The listing builds one solid part. Answer for the finished solid, in the listing's coordinates (mm). A direction names the side the tool comes from. Round coordinates to 2 decimals unless told otherwise and drop trailing zeros. Order: outer loops, then holes, each group sorted by start corner. A loop starts at its lowest first (then second) coordinate and runs counter-clockwise, first axis right, second up. Notation, with made-up numbers: (-30, 41.5) - (-18, 41.5) arc R19 cw to (-18, 47.5) - close; hole circle Ø2 at (21, -19). An arc over 180 degrees is marked (long way). Write item = value, one per line.
from build123d import *

# Parameters (mm, degrees)
SKETCH_1_R          = 95
EXTRUDE_1_DEPTH     = 50
SKETCH_2_W          = 90
SKETCH_2_H          = 100
EXTRUDE_2_DEPTH     = 150
SKETCH_3_R          = 40
CUT_EXTRUDE_1_DEPTH = 241.935676063
SHELL_1_OUTLINE_R   = 92
SHELL_1_OUTLINE_R_2 = 43
SHELL_1_DEPTH       = 47
SHELL_START         = 47
SHELL_1_2_DEPTH     = 150


# Read off the part's stored shape, not the designer's step: Оболочка1
with BuildPart() as part:
    # Эскиз1 → Бобышка-Вытянуть1 (new body)
    with BuildSketch(Plane.XY):
        Circle(SKETCH_1_R)
    extrude(amount=EXTRUDE_1_DEPTH)

    # Эскиз2 → Бобышка-Вытянуть2 (add)
    with BuildSketch(Plane.XY.offset(50)):
        Rectangle(SKETCH_2_W, SKETCH_2_H)
    extrude(amount=EXTRUDE_2_DEPTH)

    # Эскиз3 → Вырез-Вытянуть1 (cut, through all)
    with BuildSketch(Plane.XY.offset(200)):
        Circle(SKETCH_3_R)
    extrude(amount=-CUT_EXTRUDE_1_DEPTH, mode=Mode.SUBTRACT)

    # Оболочка1 outline → Оболочка1 (cut)
    with BuildSketch(Plane.XY):
        Circle(SHELL_1_OUTLINE_R)
        Circle(SHELL_1_OUTLINE_R_2, mode=Mode.SUBTRACT)
    extrude(amount=SHELL_1_DEPTH, mode=Mode.SUBTRACT)

    # Shell 1 2 outline → Shell 1 2 (cut)
    with BuildSketch(Plane.XY.offset(SHELL_START)):
        with BuildLine():
            ThreePointArc((-42, 9.219544457), (0, 43), (42, 9.219544457))
            Line((42, 9.219544457), (42, 47))
            Line((42, 47), (-42, 47))
            Line((-42, 47), (-42, 9.219544457))
        make_face()
        with BuildLine():
            Line((42, -47), (42, -9.219544457))
            ThreePointArc((42, -9.219544457), (0, -43), (-42, -9.219544457))
            Line((-42, -9.219544457), (-42, -47))
            Line((-42, -47), (42, -47))
        make_face()
    extrude(amount=SHELL_1_2_DEPTH, mode=Mode.SUBTRACT)


solid = part.part
Q1. Flat-ended cylindrical pins translate along their axes: P1, Ø4, axis at x = 50, y = -12, coming from the +Z side; P2, Ø1.5, axis at x = 43.5, z = 86, coming from the +Y side; P3, Ø2, axis at x = -71, y = -37, coming from the -Z side. Find the tip coordinate at first contact, or state that the pin passes through.
Model answer:
P1 = 50
P2 = 50
P3 = 47
Q2. Section A-A on y = 0 is taken. Determine the outline of the cut face in (x, z).
Model answer:
outline = (-95, 0) - (-92, 0) - (-92, 47) - (-43, 47) - (-43, 0) - (-40, 0) - (-40, 200) - (-45, 200) - (-45, 50) - (-95, 50) - close; (40, 0) - (43, 0) - (43, 47) - (92, 47) - (92, 0) - (95, 0) - (95, 50) - (45, 50) - (45, 200) - (40, 200) - close
Q3. Section D-D on y = -80.5 is taken. Determine the outline of the cut face in (x, z).
Model answer:
outline = (-50.45, 0) - (-44.54, 0) - (-44.54, 47) - (44.54, 47) - (44.54, 0) - (50.45, 0) - (50.45, 50) - (-50.45, 50) - close
Q4. Find the intervals of material crossed by line 1 (Y direction, x = 0, z = 100.5); line 2 (Y direction, x = 0, z = 24); line 3 (X direction, y = 17, z = 119), in increasing order. Write a range as from..to.
Model answer:
line_1 = -50..-47, -43..-40, 40..43, 47..50
line_2 = -95..-92, -43..-40, 40..43, 92..95
line_3 = -45..-42, -39.5..-36.21, 36.21..39.5, 42..45
Q5. For faces 1 (the face through (-45, -1, 124)), 2 (the face through (-8.67, -39.05, 101.4)), 3 (the face through (-1, -50, 124)), 4 (the face through (1, 47, 121)), 5 (the face through (38, -13, 0)), determine the directions among +Z, -Z, +X, -X, +Y, -Y from which every point of the face is accessible in a straight line to the end or side of a thin tool.
Model answer:
face_1 = +Z, -X, +Y, -Y
face_2 = +Z, -Z
face_3 = +Z, +X, -X, -Y
face_4 = -Z
face_5 = -Z, +X, -X, +Y, -Y
Q6. Section B-B on x = 0 is taken. Determine the outline of the cut face in (y, z).
Model answer:
outline = (-95, 0) - (-92, 0) - (-92, 47) - (-47, 47) - (-47, 197) - (-43, 197) - (-43, 0) - (-40, 0) - (-40, 200) - (-50, 200) - (-50, 50) - (-95, 50) - close; (40, 0) - (43, 0) - (43, 197) - (47, 197) - (47, 47) - (92, 47) - (92, 0) - (95, 0) - (95, 50) - (50, 50) - (50, 200) - (40, 200) - close
Q7. Section C-C on z = 183.5 is taken. Determine the outline of the cut face in (x, y), then the cut area to 3 significant figures.
Model answer:
outline = (-45, -50) - (45, -50) - (45, 50) - (-45, 50) - close; hole (-42, -47) - (42, -47) - (42, -9.22) arc R43 cw to (-42, -9.22) - close; hole (-42, 9.22) arc R43 cw to (42, 9.22) - (42, 47) - (-42, 47) - close; hole circle Ø80 at (0, 0)
area = 1,860 mm^2
Q8. Determine the mould class of faces 6 (the face through (-42, -28, 121)), 7 (the face through (45, -1, 124)), 8 (the face through (-1, 50, 124)) for opening direction Y: released by +Y, released by -Y, zero draft, split by the parting line, or undercut.
Model answer:
face_6 = undercut
face_7 = zero draft
face_8 = released by +Y
